```python
from build123d import *

# Parameters (mm, degrees)
AUFSATZ_LINEAR_AUSTRAGEN1_DEPTH      = 80
AUFSATZ_LINEAR_AUSTRAGEN2_DEPTH      = 8
SKIZZE3_W                            = 49
SKIZZE3_H                            = 50
AUFSATZ_LINEAR_AUSTRAGEN4_DEPTH      = 0.5
AUFSATZ_LINEAR_AUSTRAGEN4_DEPTH_BACK = 0.1
DURCHGANGSLOCH_F_R_M81_D             = 9


with BuildPart() as part:
    # Skizze1 → Aufsatz-Linear austragen1 (new body)
    with BuildSketch(Plane(origin=(0, 0, 0), x_dir=(1, 0, 0), z_dir=(0, 1, 0))):
        with BuildLine():
            Line((-154.797525399, -7.583806671), (-154.797525399, -10.583806671))
            Line((-154.797525399, -10.583806671), (-2.797525399, -10.583806671))
            ThreePointArc((-2.797525399, -10.583806671), (-2.090418618, -10.290913452), (-1.797525399, -9.583806671))
            Line((-1.797525399, -9.583806671), (-1.797525399, 94.416193329))
            Line((-1.797525399, 94.416193329), (-4.797525399, 94.416193329))
            Line((-4.797525399, 94.416193329), (-4.797525399, -6.583806671))
            ThreePointArc((-4.797525399, -6.583806671), (-5.090418618, -7.290913452), (-5.797525399, -7.583806671))
            Line((-5.797525399, -7.583806671), (-154.797525399, -7.583806671))
        make_face()
    extrude(amount=AUFSATZ_LINEAR_AUSTRAGEN1_DEPTH)

    # Skizze2 → Aufsatz-Linear austragen2 (add)
    with BuildSketch(Plane.XY.offset(10.583806671)):
        with BuildLine():
            Line((-45.297525399, -2.5), (-130.297525399, -2.5))
            ThreePointArc((-130.297525399, -2.5), (-132.065292352, -1.767766953), (-132.797525399, 0))
            Line((-132.797525399, 0), (-132.797525399, 80))
            ThreePointArc((-132.797525399, 80), (-132.065292352, 81.767766953), (-130.297525399, 82.5))
            Line((-130.297525399, 82.5), (-45.297525399, 82.5))
            ThreePointArc((-45.297525399, 82.5), (-43.529758446, 81.767766953), (-42.797525399, 80))
            Line((-42.797525399, 80), (-42.797525399, 0))
            ThreePointArc((-42.797525399, 0), (-43.529758446, -1.767766953), (-45.297525399, -2.5))
        make_face()
    extrude(amount=AUFSATZ_LINEAR_AUSTRAGEN2_DEPTH)


with BuildPart() as body_2:
    # Skizze3 → Aufsatz-Linear austragen4 (new body, two sides)
    with BuildSketch(Plane.XY.offset(18.583806671)) as aufsatz_linear_austragen4_sk:
        with Locations((-88.297525399, 39.5)):
            Rectangle(SKIZZE3_W, SKIZZE3_H)
    extrude(amount=AUFSATZ_LINEAR_AUSTRAGEN4_DEPTH)
    extrude(aufsatz_linear_austragen4_sk.sketch, amount=-AUFSATZ_LINEAR_AUSTRAGEN4_DEPTH_BACK)


with BuildPart() as part_1:
    add(part.part)

    # Kombinieren1: cut body 2
    add(body_2.part, mode=Mode.SUBTRACT)

    # Durchgangsloch für M81 (through all)
    with Locations(Plane(origin=(-1.797525399, 0, 0), x_dir=(0, 0, -1), z_dir=(1, 0, 0))):
        with Locations((37.416193329, 40)):
            Hole(DURCHGANGSLOCH_F_R_M81_D / 2)


solid = part_1.part
```
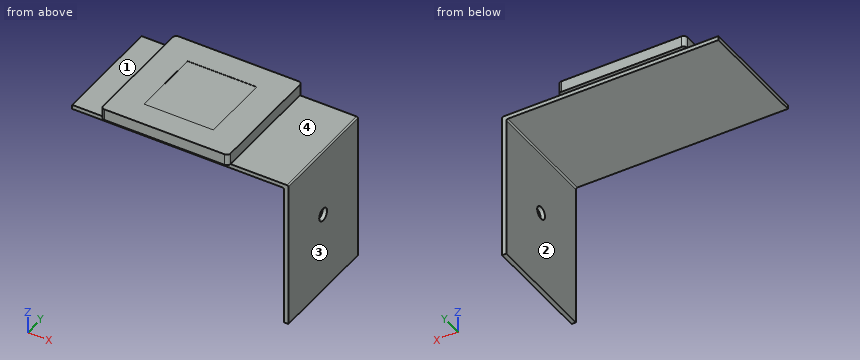
The listing builds one solid part. Answer for the finished solid, in the listing's coordinates (mm). Face numbers are marked on the shaded views. A direction names the side the tool comes from. Coordinates: 2 decimals unless noted, no trailing zeros. Write each loop counter-clockwise with the first axis right and the second up, starting at its lowest first coordinate (ties: lowest second). Pieces come first, ordered by that corner, then holes. Notation, with made-up numbers: (52.5, 78.25) - (82.5, 78.25) arc R24 cw to (82.5, 104.25) - close; hole circle Ø10 at (63, 19.25). An arc over 180 degrees is marked (long way). Return JSON: item names as keys, results as strings. Group by question number.
Q1. The part is cut by section A-A on y = 40. Write down the section's boundary in (x, z), and give its area (3 significant figures).
Q2. Find the intervals of material crossed by line 1 along X through (y, z) = (54, -63.5); line 2 along Z through (x, y) = (-126, 67); line 3 along Z through (x, y) = (-143.5, 24), in increasing order. Write a range as [from, to].
Q3. The part is cut by section C-C on x = -106.5. Write down the section's boundary in (y, z), and give its area (3 significant figures).
Q4. Which of the six approach directions +Z, -Z, +X, -X, +Y, -Y give full straight-line access (tool end or side, diameter ignored) to the marked faces 1, 2, 3 and 4?
Q5. The part is cut by section D-D on z = -84.5. Write down the section's boundary in (x, y).
Q6. Flat-ended cylindrical pins translate along their axes: pin 1 Ø9 at (y, z) = (42.5, 13) entering from -X; pin 2 Ø2 at (y, z) = (59.5, -26.5) entering from -X; pin 3 Ø8 at (x, y) = (-99.5, 28.5) entering from +Z; pin 4 Ø3 at (x, y) = (-85, 81) entering from -Z. Find the tip coordinate at first contact, or state that the pin passes through.
Q7. The part is cut by section B-B on y = 6. Write down the section's boundary in (x, z), and give its area (4 significant figures).
Evaluation:
{
 "1": {"outline": "(-154.8, 7.58) - (-5.8, 7.58) arc R1 cw to (-4.8, 6.58) - (-4.8, -32.92) - (-1.8, -32.92) - (-1.8, 9.58) arc R1 ccw to (-2.8, 10.58) - (-42.8, 10.58) - (-42.8, 18.58) - (-63.8, 18.58) - (-63.8, 18.48) - (-112.8, 18.48) - (-112.8, 18.58) - (-132.8, 18.58) - (-132.8, 10.58) - (-154.8, 10.58) - close; (-4.8, -94.42) - (-1.8, -94.42) - (-1.8, -41.92) - (-4.8, -41.92) - close", "area": "1,450 mm2"},
 "2": {"line 1": "x = [-4.8, -1.8]", "line 2": "z = [7.58, 18.58]", "line 3": "z = [7.58, 10.58]"},
 "3": {"outline": "(-2.5, 10.58) - (0, 10.58) - (0, 7.58) - (80, 7.58) - (80, 10.58) - (82.5, 10.58) - (82.5, 18.58) - (64.5, 18.58) - (64.5, 18.48) - (14.5, 18.48) - (14.5, 18.58) - (-2.5, 18.58) - close", "area": "915 mm2"},
 "4": {"face 1": "+Z, -X, +Y, -Y", "face 2": "-Z, -X, +Y, -Y", "face 3": "+Z, -Z, +X, +Y, -Y", "face 4": "+Z, +X, +Y, -Y"},
 "5": {"outline": "(-4.8, 0) - (-1.8, 0) - (-1.8, 80) - (-4.8, 80) - close"},
 "6": {"pin 1": "stops at x = -154.8", "pin 2": "stops at x = -4.8", "pin 3": "stops at z = 18.48", "pin 4": "stops at z = 7.58"},
 "7": {"outline": "(-154.8, 7.58) - (-5.8, 7.58) arc R1 cw to (-4.8, 6.58) - (-4.8, -94.42) - (-1.8, -94.42) - (-1.8, 9.58) arc R1 ccw to (-2.8, 10.58) - (-42.8, 10.58) - (-42.8, 18.58) - (-132.8, 18.58) - (-132.8, 10.58) - (-154.8, 10.58) - close", "area": "1,485 mm2"}
}
